Check sheet for the modelled part. Datum: model origin and axes. Units: mm. Face numbers are marked on the shaded views. A direction names the side the tool comes from. Round coordinates to 2 decimals unless told otherwise and drop trailing zeros. Write each loop counter-clockwise with the first axis right and the second up, starting at its lowest first coordinate (ties: lowest second). Pieces come first, ordered by that corner, then holes.
Item 1: Material ranges on line 1 (Y direction, x = 66.5, z = -32); line 2 (Y direction, x = 54.5, z = -7); line 3 (Z direction, x = -16.5, y = 40), recorded low to high.
Item 2: Cross-section at C-C on x = 93. Enter the section's corners in (y, z), plus the area to 3 significant figures.
Item 3: Tool access check on the marked faces 5, 6, 7, 8 and 9. Record the directions out of +Z, -Z, +X, -X, +Y, -Y that give a thin tool (end or side, any length) a straight path to the whole face; none if there is none.
Item 4: Cross-section at D-D on z = -58.5. Enter the section's corners in (x, y).
Item 5: Cross-section at B-B on y = 48.5. Enter the section's corners in (x, z), plus the area to 3 significant figures.
Item 6: Cross-section at A-A on x = 58.5. Enter the section's corners in (y, z), plus the area to 3 significant figures.
Item 7: Go/stop test with flat-tipped pins: pin 1 Ø10 at (x, y) = (112.5, 43.5) entering from +Z; pin 2 Ø6 at (x, y) = (23.5, 115) entering from -Z; pin 3 Ø7.5 at (x, z) = (93.5, -31.5) entering from +Y; pin 4 Ø6 at (x, y) = (4, 40) entering from -Z. Record where each tip stops, or that it passes through.
Item 8: Release check for a two-part mould opening along Y. For the marked faces 1, 2, 3 and 4 record: +Y half, -Y half, draft (parallel to the pull), parting line (faces both ways), or undercut.
from build123d import *

# Parameters (mm, degrees)
BOSS_EXTRU_1_DEPTH      = 64
BOSS_EXTRU_2_DEPTH      = 19
ENL_V_MAT_EXTRU_1_REACH = 212.704
ESQUISSE3_R             = 9.5
ENL_V_MAT_EXTRU_2_DEPTH = 6
ESQUISSE5_R             = 19.5
ENL_V_MAT_EXTRU_3_DEPTH = 12
ESQUISSE6_W             = 22
ESQUISSE6_H             = 56
ENL_V_MAT_EXTRU_4_DEPTH = 6
BOSS_EXTRU_3_DEPTH      = 70
ESQUISSE9_W             = 40
ESQUISSE9_H             = 30.5
ENL_V_MAT_EXTRU_5_DEPTH = 189.718687482
ESQUISSE10_R            = 7.5
ENL_V_MAT_EXTRU_6_DEPTH = 168.72147449
CONG_1_R                = 10


with BuildPart() as part:
    # Esquisse1 → Boss.-Extru.1 (new body)
    with BuildSketch(Plane.XY):
        Polygon((0, 0), (-45, 77.942286341), (-0.832704407, 103.442286341), (8.667295593, 86.987803669), (-19.045517328, 70.987803669), (10.969655115, 19), (140, 19), (140, 0), align=None)
    extrude(amount=-BOSS_EXTRU_1_DEPTH)

    # Esquisse2 → Boss.-Extru.2 (add)
    with BuildSketch(Plane(origin=(-45, 77.942286341, 0), x_dir=(0.8660254037844398, 0.49999999999999806, 0), z_dir=(-0.499999999999998, 0.8660254037844397, 0))):
        with BuildLine():
            Line((51, 64), (51, 0))
            ThreePointArc((51, 0), (83, 32), (51, 64))
        make_face()
    extrude(amount=-BOSS_EXTRU_2_DEPTH)

    # Esquisse3 → Enlèv. mat.-Extru.1 (cut, up to next)
    with BuildSketch(Plane(origin=(-45, 77.942286341, 0), x_dir=(0.8660254037844398, 0.49999999999999806, 0), z_dir=(-0.499999999999998, 0.8660254037844397, 0)), mode=Mode.PRIVATE) as enl_v_mat_extru_1_sk1:
        with Locations(Location((51, 32, 0), (0, 0, 180))):
            Circle(ESQUISSE3_R)
    enl_v_mat_extru_1_tool1 = extrude(enl_v_mat_extru_1_sk1.sketch, amount=-ENL_V_MAT_EXTRU_1_REACH, mode=Mode.PRIVATE) & part.part
    add(enl_v_mat_extru_1_tool1.solids().sort_by_distance((-0.832704, 103.442286, -32))[0], mode=Mode.SUBTRACT)

    # Esquisse4 → Enlèv. mat.-Extru.2 (cut)
    with BuildSketch(Plane(origin=(-45, 77.942286341, 0), x_dir=(0.8660254037844398, 0.49999999999999806, 0), z_dir=(-0.499999999999998, 0.8660254037844397, 0))):
        with BuildLine():
            Line((0, 43), (81.049958403, 43))
            ThreePointArc((81.049958403, 43), (83, 32), (81.049958403, 21))
            Line((81.049958403, 21), (0, 21))
            Line((0, 21), (0, 43))
        make_face()
    extrude(amount=-ENL_V_MAT_EXTRU_2_DEPTH, mode=Mode.SUBTRACT)

    # Esquisse5 → Enlèv. mat.-Extru.3 (cut)
    with BuildSketch(Plane(origin=(-45, 77.942286341, 0), x_dir=(0.8660254037844398, 0.49999999999999806, 0), z_dir=(-0.499999999999998, 0.8660254037844397, 0))):
        with Locations(Location((51, 32, 0), (0, 0, 180))):
            Circle(ESQUISSE5_R)
    extrude(amount=-ENL_V_MAT_EXTRU_3_DEPTH, mode=Mode.SUBTRACT)

    # Esquisse6 → Enlèv. mat.-Extru.4 (cut)
    with BuildSketch(Plane(origin=(0, 0, 0), x_dir=(0, 0, 1), z_dir=(-0.8660254037844398, -0.49999999999999806, 0))):
        with Locations((-32, 62)):
            Rectangle(ESQUISSE6_W, ESQUISSE6_H)
    extrude(amount=-ENL_V_MAT_EXTRU_4_DEPTH, mode=Mode.SUBTRACT)

    # Esquisse8 → Boss.-Extru.3 (add)
    with BuildSketch(Plane(origin=(125, 0, 0), x_dir=(0, 0, -1), z_dir=(1, 0, 0))):
        with BuildLine():
            Line((19.5, 19), (19.5, 44))
            ThreePointArc((19.5, 44), (32, 56.5), (44.5, 44))
            Line((44.5, 44), (44.5, 19))
            Line((44.5, 19), (19.5, 19))
        make_face()
    extrude(amount=-BOSS_EXTRU_3_DEPTH)

    # Esquisse9 → Enlèv. mat.-Extru.5 (cut, through all)
    with BuildSketch(Plane.XY.offset(-19.5)):
        with Locations((90, 41.25)):
            Rectangle(ESQUISSE9_W, ESQUISSE9_H)
    extrude(amount=-ENL_V_MAT_EXTRU_5_DEPTH, mode=Mode.SUBTRACT)

    # Esquisse10 → Enlèv. mat.-Extru.6 (cut, through all)
    with BuildSketch(Plane.ZY.offset(-55)):
        with Locations((-32, 44)):
            Circle(ESQUISSE10_R)
    extrude(amount=-ENL_V_MAT_EXTRU_6_DEPTH, mode=Mode.SUBTRACT)

    # Congé1
    cong_1_edges = [part.edges().sort_by_distance(p)[0] for p in [
        (-19.045517328, 70.987803669, -32),
        (10.969655115, 19, -32),
    ]]
    fillet(cong_1_edges, radius=CONG_1_R)


solid = part.part
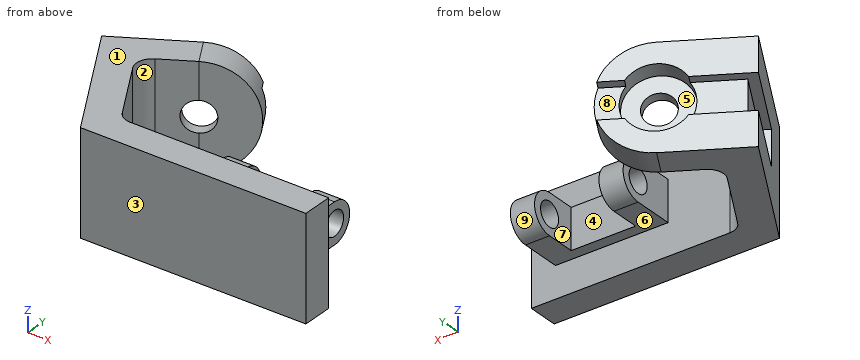
Response values:
1. line 1: y = 0 to 36.5, 51.5 to 56.5
1. line 2: y = 0 to 19
1. line 3: z = -64 to -43, -21 to 0
2. outline: (0, -64) - (19, -64) - (19, -44.5) - (26, -44.5) - (26, -19.5) - (19, -19.5) - (19, 0) - (0, 0) - close
2. area: 1,390 mm2
3. face 5: none
3. face 6: -Z, +X, +Y
3. face 7: +Z, -Z, +Y
3. face 8: -X, +Y
3. face 9: +X, +Y
4. outline: (-45, 77.94) - (0, 0) - (140, 0) - (140, 19) - (16.74, 19) arc R10 cw to (8.08, 24) - (-14.05, 62.33) arc R10 cw to (-10.39, 75.99) - (24.2, 95.96) - (14.7, 112.41) - close
5. outline: (-28, -64) - (-6.06, -64) - (-6.06, 0) - (-28, 0) - (-28, -21) - (-21.07, -21) - (-21.07, -43) - (-28, -43) - close; (55, -43.66) - (70, -43.66) - (70, -38) - (55, -38) - close; (55, -26) - (70, -26) - (70, -20.34) - (55, -20.34) - close; (110, -43.66) - (125, -43.66) - (125, -38) - (110, -38) - close; (110, -26) - (125, -26) - (125, -20.34) - (110, -20.34) - close
5. area: 1,590 mm2
6. outline: (0, -64) - (19, -64) - (19, -44.5) - (44, -44.5) arc R12.5 ccw to (44, -19.5) - (19, -19.5) - (19, 0) - (0, 0) - close; hole circle Ø15 at (44, -32)
6. area: 1,910 mm2
7. pin 1: stops at z = -19.5
7. pin 2: stops at z = -53.33
7. pin 3: stops at y = 26
7. pin 4: passes through
8. face 1: draft
8. face 2: undercut
8. face 3: -Y half
8. face 4: +Y half
